The model under review builds one solid part; all positions refer to its coordinate system, in mm. A direction names the side the tool comes from. Coordinates: 2 decimals unless noted, no trailing zeros. Write each loop counter-clockwise with the first axis right and the second up, starting at its lowest first coordinate (ties: lowest second). Pieces come first, ordered by that corner, then holes. Notation, with made-up numbers: M -23,69.25 L 13,69.25 A16 ccw 13,92.25 Z; hole C -35,-23 d6. An arc over 180 degrees is marked long. Answer as CSV lines item,"result". Start each with the question number.
Autodesk Inventor part; units mm, degrees
ref_plane "YZ Plane" through (0, 0, 0) normal (1, 0, 0) x (0, 1, 0)
ref_plane "XZ Plane" through (0, 0, 0) normal (0, 1, 0) x (-1, 0, 0)
ref_plane "XY Plane" through (0, 0, 0) normal (0, 0, 1) x (1, 0, 0)
sketch "草图1" plane through (0, 0, 0) normal (0, 0, 1) x (1, 0, 0)
  line L0 (2.5, -9.5) -> (-2.5, -9.5)
  line L1 (-2.5, -9.5) -> (-2.5, 9.5)
  line L2 (-2.5, 9.5) -> (2.5, 9.5)
  line L3 (2.5, 9.5) -> (2.5, -9.5)
  line L4 (2.5, -9.5) -> (-2.5, 9.5) construction
  line L5 (-2.5, -9.5) -> (2.5, 9.5) construction
  point P0 (0, 0)
  dimension "d0" = 5
  dimension "d1" = 19
extrude "拉伸1" add sketch "草图1" along normal blind 3
sketch "草图2" plane through (0, 0, 3) normal (0, 0, 1) x (1, 0, 0)
  line L0 (2.5, 9.5) -> (-2.5, 9.5)
  line L1 (-2.5, -9.5) -> (2.5, -9.5)
  line L2 (-2.5, 9.5) -> (-1.5, 9.5)
  line L3 (-1.5, 9.5) -> (-1.5, -9.5)
  line L4 (-1.5, -9.5) -> (-2.5, -9.5)
  line L5 (-2.5, -9.5) -> (-2.5, 9.5)
  point P0 (0, 0)
  dimension "d4" = 1
extrude "拉伸2" add sketch "草图2" along normal blind 1
sketch "草图3" plane through (-2.5, -9.5, 0) normal (-1, 0, 0) x (0, 0, 1)
  line L0 (0.9436, 15) -> (0.9436, 3) construction
  line L1 (-0.0564, 15) -> (-0.0564, 3)
  line L2 (1.9436, 3) -> (1.9436, 15)
  arc A0 (1.9436, 15) -> (-0.0564, 15) centre (0.9436, 15) ccw
  arc A1 (-0.0564, 3) -> (1.9436, 3) centre (0.9436, 3) ccw
  line L3 (0, 19) -> (4, 19)
  point P0 (0, 9.5)
  point P1 (0.9436, 9)
  point P2 (0.9436, 16)
  point P3 (0.9436, 2)
  dimension "d7" = 2
  dimension "d8" = 14
  dimension "d9" = 3
extrude "拉伸3" add sketch "草图3" along normal blind 3
properties part number "指纹识别"
1) To check wall thickness, follow line 1 (Z direction, x = -3.5, y = 0); line 2 (X direction, y = 6.75, z = 3.7); line 3 (X direction, y = -7.75, z = 1.9). State the ranges of each line that lie inside material, in increasing order. Write a range as [from, to].
2) Take a section at D-D on y = -1. Give the boundary of the cut face in (x, z).
3) Tool access review of faces 1 (the flat face through (0, 0, 0)), 2 (the flat face through (-1.5, 0.1, 3.5)), 3 (the flat face through (-4, -1, 1.944)), 4 (the cylindrical face through (-4, -7.5, 1)), 5 (the cylindrical face through (-4, 6.5, 0.9)): name each direction out of +Z, -Z, +X, -X, +Y, -Y from which nothing blocks a thin tool from reaching the whole face with its end or side.
4) Take a section at A-A on y = 6.75. Give the boundary of the cut face in (x, z).
5) Take a section at C-C on x = -0.5. Give the boundary of the cut face in (y, z).
6) Take a section at B-B on z = 2.45. Give the boundary of the cut face in (x, y), and give its area (3 significant figures).
7) Clearance check with flat-ended pins moving along their axes: pin 1 Ø1.2 at (x, y) = (1, -3) entering from +Z; pin 2 Ø4 at (x, y) = (0.5, -1.5) entering from -Z; pin 3 Ø3.5 at (x, y) = (-4.5, -2) entering from +Z. State where each tip first meets the part, or that it passes through.
Results:
1,line 1,"z = [-0.06, 1.94]"
1,line 2,"x = [-2.5, -1.5]"
1,line 3,"x = [-2.5, 2.5]"
2,outline,"M -5.5,-0.06 L -2.5,-0.06 L -2.5,0 L 2.5,0 L 2.5,3 L -1.5,3 L -1.5,4 L -2.5,4 L -2.5,1.94 L -5.5,1.94 Z"
3,face 1,"-Z, +X, +Y, -Y"
3,face 2,"+Z, +X, +Y, -Y"
3,face 3,"+Z, -X, +Y, -Y"
3,face 4,"-X, -Y"
3,face 5,"-X, +Y"
4,outline,"M -2.5,0 L 2.5,0 L 2.5,3 L -1.5,3 L -1.5,4 L -2.5,4 Z"
5,outline,"M -9.5,0 L 9.5,0 L 9.5,3 L -9.5,3 Z"
6,outline,"M -2.5,-9.5 L 2.5,-9.5 L 2.5,9.5 L -2.5,9.5 Z"
6,area,"95.0 mm²"
7,pin 1,"stops at z = 3"
7,pin 2,"stops at z = 0"
7,pin 3,"stops at z = 1.94"
